Can you work these out from the model? Positions are in its coordinate system, mm. Give positions to 0.01 mm unless a question says otherwise; leave off trailing zeros. Write each loop counter-clockwise with the first axis right and the second up, starting at its lowest first coordinate (ties: lowest second). Pieces come first, ordered by that corner, then holes.
1. Suppose I cut it at B-B (x = 42). Please give me the cut outline in (y, z), and give its area (3 significant figures).
2. If I drill on probe 1 along Z at (x, y) = (42, -1.25); probe 2 along X at (y, z) = (-0.95, -23); probe 3 along Z at (x, y) = (-40, -1.55), over which ranges is the centre line in solid material (lowest first)?
3. Suppose I cut it at A-A (z = 22). Please give me the cut outline in (x, y).
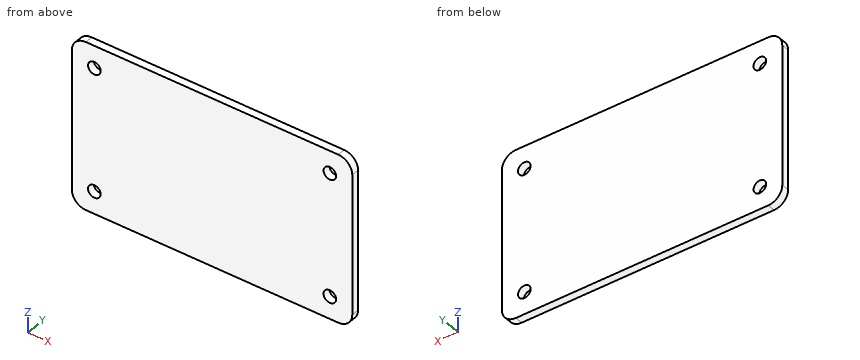
```python
from build123d import *

# Parameters (mm, degrees)
F0_R     = 2.25
F1_DEPTH = 2.8


with BuildPart() as f1:
    # F0 (on Front) → F1 (new body)
    with BuildSketch(Plane.XZ):
        with BuildLine():
            Line((-45, -30), (45, -30))
            ThreePointArc((45, -30), (48.535534, -28.535534), (50, -25))
            Line((50, -25), (50, 25))
            ThreePointArc((50, 25), (48.535534, 28.535534), (45, 30))
            Line((45, 30), (-45, 30))
            ThreePointArc((-45, 30), (-48.535534, 28.535534), (-50, 25))
            Line((-50, 25), (-50, -25))
            ThreePointArc((-50, -25), (-48.535534, -28.535534), (-45, -30))
        make_face()
        with BuildLine():
            ThreePointArc((45, 27.000001), (46.414214, 26.414214), (47.000001, 25))
            Line((47.000001, 25), (47.000001, -25))
            ThreePointArc((47.000001, -25), (46.414214, -26.414214), (45, -27.000001))
            Line((45, -27.000001), (-45, -27.000001))
            ThreePointArc((-45, -27.000001), (-46.414214, -26.414214), (-47.000001, -25))
            Line((-47.000001, -25), (-47.000001, 25))
            ThreePointArc((-47.000001, 25), (-46.414214, 26.414214), (-45, 27.000001))
            Line((-45, 27.000001), (45, 27.000001))
        make_face(mode=Mode.SUBTRACT)
        with BuildLine():
            Line((47.000001, -25), (47.000001, 25))
            ThreePointArc((47.000001, 25), (46.414214, 26.414214), (45, 27.000001))
            Line((45, 27.000001), (-45, 27.000001))
            ThreePointArc((-45, 27.000001), (-46.414214, 26.414214), (-47.000001, 25))
            Line((-47.000001, 25), (-47.000001, -25))
            ThreePointArc((-47.000001, -25), (-46.414214, -26.414214), (-45, -27.000001))
            Line((-45, -27.000001), (45, -27.000001))
            ThreePointArc((45, -27.000001), (46.414214, -26.414214), (47.000001, -25))
        make_face()
        with Locations((-42, -22)):
            Circle(F0_R, mode=Mode.SUBTRACT)
        with Locations((42, -22)):
            Circle(F0_R, mode=Mode.SUBTRACT)
        with Locations((-42, 22)):
            Circle(F0_R, mode=Mode.SUBTRACT)
        with Locations((42, 22)):
            Circle(F0_R, mode=Mode.SUBTRACT)
    extrude(amount=F1_DEPTH)


solid = f1.part
```
Checks:
1. outline: (-2.8, -30) - (0, -30) - (0, -24.25) - (-2.8, -24.25) - close; (-2.8, -19.75) - (0, -19.75) - (0, 19.75) - (-2.8, 19.75) - close; (-2.8, 24.25) - (0, 24.25) - (0, 30) - (-2.8, 30) - close
1. area: 143 mm2
2. probe 1: z = -30 to -24.25, -19.75 to 19.75, 24.25 to 30
2. probe 2: x = -50 to -44.02, -39.98 to 39.98, 44.02 to 50
2. probe 3: z = -30 to -23.03, -20.97 to 20.97, 23.03 to 30
3. outline: (-50, -2.8) - (-44.25, -2.8) - (-44.25, 0) - (-50, 0) - close; (-39.75, -2.8) - (39.75, -2.8) - (39.75, 0) - (-39.75, 0) - close; (44.25, -2.8) - (50, -2.8) - (50, 0) - (44.25, 0) - close
